The model under review builds one solid part; all positions refer to its coordinate system, in mm. A direction names the side the tool comes from. Round coordinates to 2 decimals unless told otherwise and drop trailing zeros. Write each loop counter-clockwise with the first axis right and the second up, starting at its lowest first coordinate (ties: lowest second). Pieces come first, ordered by that corner, then holes.
Item 1: Draft analysis for pull direction X (two halves, no side actions). For faces 3 (the face through (-2, 0, -32)), 4 (the face through (-21.623, -2.465, -175.575)), 5 (the face through (-4.51, -2.46, -138.88)), 6 (the face through (-126.15, -2.465, -55.314)), state which applies: +X half, -X half, draft (parallel to the pull), parting line (faces both ways), or undercut.
Item 2: Add section B-B (y = -3.9). State how many separate pieces and enclosed holes the cut face has, plus the area to 3 significant figures.
Item 3: To check wall thickness, follow L1, parallel to X at y = -1.05, z = -132.5; L2, parallel to X at y = -2.7, z = -132; L3, parallel to Z at x = 4.5, y = -4.1. State the ranges of each line that lie inside material, in increasing order.
Item 4: Machinability: for faces 1 (the face through (125.83, -2.46, -55.99)), 2 (the face through (20.94, -2.46, -175.7)), which of the approach directions +Z, -Z, +X, -X, +Y, -Y give a long, thin tool a straight path to every point of the face, cutting with its end or side? Answer none if there is none.
Item 5: Add section A-A (z = -162). Give the boundary of the cut face in (x, y), plus the area to 3 significant figures.
Item 6: Clearance check with flat-ended pins moving along their axes: pin 1 Ø2 at (x, y) = (55.5, -2.5) entering from +Z; pin 2 Ø1.5 at (y, z) = (-3, -121.5) entering from -X; pin 3 Ø2.5 at (y, z) = (-3.5, 6) entering from -X. State where each tip first meets the part, or that it passes through.
```python
from build123d import *

# Parameters (mm, degrees)
F0_R     = 1.6
F0_R_2   = 1.5
F1_DEPTH = 5


with BuildPart() as f1:
    # F0 (on Front) → F1 (new body)
    with BuildSketch(Plane.XZ):
        with BuildLine():
            Line((0, -105.5724638663), (0, -98.9320270717))
            Line((0, -98.9320270717), (0, -87.6365141757))
            Line((0, -87.6365141757), (-49.5, -87.6365141757))
            Line((-49.5, -87.6365141757), (-49.5, -59.3522429283))
            Line((-49.5, -59.3522429283), (0, -59.3522429283))
            Line((0, -59.3522429283), (0, 98.9320270717))
            add(Edge.make_bspline(
                [(-146.2381845713, 48.9320270717), (-143.2091262015, 68.9096288331), (-135.5852518703, 119.1915008468), (-50.9865840375, 106.55056484), (0, 98.9320270717)],
                knots=[0, 0, 0, 0, 0.3973122114, 1, 1, 1, 1], degree=3))
            Line((-146.2381845713, 48.9320270717), (-125, 48.9320270717))
            Line((-125, 48.9320270717), (-76.2381845713, 48.9320270717))
            Line((-76.2381845713, 48.9320270717), (-76.2381845713, -34.5724638663))
            Line((-76.2381845713, -34.5724638663), (-141.8916900928, -34.5724638663))
            ThreePointArc((-141.8916900928, -34.5724638663), (-125.9898971587, -55.6502114599), (-119.7161859861, -81.2974142364))
            Line((-119.7161859861, -81.2974142364), (-125, -98.9320270717))
            Line((-125, -98.9320270717), (-125, -142.2410042337))
            ThreePointArc((-125, -142.2410042337), (-123.6989053151, -148.3516501216), (-120.0213342443, -153.4022254914))
            Line((-120.0213342443, -153.4022254914), (-103.4289673704, -168.3000265931))
            ThreePointArc((-103.4289673704, -168.3000265931), (-65.4068612322, -117.6788317827), (-43.2242829938, -176.9757047349))
            ThreePointArc((-43.2242829938, -176.9757047349), (-44.2540337338, -178.1193368484), (-45.3315999714, -179.2180324392))
            ThreePointArc((-45.3315999714, -179.2180324392), (-21.2811980726, -175.6350274134), (0, -187.3981207609))
            Line((0, -187.3981207609), (0, -179.2180324392))
            Line((0, -179.2180324392), (0, -145.0724638663))
            ThreePointArc((0, -145.0724638663), (-1.0813916472, -144.6119791886), (-1.4988309156, -143.51325334))
            ThreePointArc((-1.4988309156, -143.51325334), (-16.4544826719, -134.0724638663), (-17.1526203097, -116.4000947784))
            ThreePointArc((-17.1526203097, -116.4000947784), (-17.7535207776, -114.3224638663), (-15.6537893941, -113.8040434806))
            ThreePointArc((-15.6537893941, -113.8040434806), (-8.843076746, -107.755805647), (0, -105.5724638663))
        make_face()
        with Locations((-59.6421356237, -73.494378552)):
            Circle(F0_R, mode=Mode.SUBTRACT)
        with BuildLine():
            ThreePointArc((-70.2381845713, -6.0724638663), (-71.298844743, -3.5118036945), (-68.7381845713, -4.5724638663))
            ThreePointArc((-68.7381845713, -4.5724638663), (-69.1775243995, -5.6331240381), (-70.2381845713, -6.0724638663))
        make_face(mode=Mode.SUBTRACT)
        with Locations((-64.1868777356, -4.5724638663)):
            Circle(F0_R_2, mode=Mode.SUBTRACT)
        with Locations((-58.2381845713, -4.5724638663)):
            Circle(F0_R_2, mode=Mode.SUBTRACT)
        with Locations((-70.2381845713, 24.4275361337)):
            Circle(F0_R_2, mode=Mode.SUBTRACT)
        with Locations((-64.2381845713, 24.4275361337)):
            Circle(F0_R_2, mode=Mode.SUBTRACT)
        with Locations((-58.2381845713, 24.4275361337)):
            Circle(F0_R_2, mode=Mode.SUBTRACT)
        with BuildLine():
            Line((0, -87.6365141757), (0, -98.9320270717))
            Line((0, -98.9320270717), (0, -105.5724638663))
            ThreePointArc((0, -105.5724638663), (8.843076746, -107.755805647), (15.6537893941, -113.8040434806))
            ThreePointArc((15.6537893941, -113.8040434806), (17.178692615, -113.7588733828), (17.9544826719, -115.0724638663))
            ThreePointArc((17.9544826719, -115.0724638663), (17.738462122, -115.8479616237), (17.1526203097, -116.4000947784))
            ThreePointArc((17.1526203097, -116.4000947784), (18.5324011651, -120.3831790756), (19, -124.5724638663))
            ThreePointArc((19, -124.5724638663), (13.9548878067, -137.4666915013), (1.4988309156, -143.51325334))
            ThreePointArc((1.4988309156, -143.51325334), (1.4997077004, -143.542852833), (1.5, -143.5724638663))
            ThreePointArc((1.5, -143.5724638663), (1.0606601718, -144.6331240381), (0, -145.0724638663))
            Line((0, -145.0724638663), (0, -179.2180324392))
            Line((0, -179.2180324392), (0, -187.3981207609))
            ThreePointArc((0, -187.3981207609), (21.2811980726, -175.6350274134), (45.3315999714, -179.2180324392))
            ThreePointArc((45.3315999714, -179.2180324392), (44.2540337338, -178.1193368484), (43.2242829938, -176.9757047349))
            ThreePointArc((43.2242829938, -176.9757047349), (65.4068612322, -117.6788317827), (103.4289673704, -168.3000265931))
            Line((103.4289673704, -168.3000265931), (120.0213342443, -153.4022254914))
            ThreePointArc((120.0213342443, -153.4022254914), (123.6989053151, -148.3516501216), (125, -142.2410042337))
            Line((125, -142.2410042337), (125, -98.9320270717))
            Line((125, -98.9320270717), (119.7161859861, -81.2974142364))
            ThreePointArc((119.7161859861, -81.2974142364), (125.9898971587, -55.6502114599), (141.8916900928, -34.5724638663))
            Line((141.8916900928, -34.5724638663), (76.2381845713, -34.5724638663))
            Line((76.2381845713, -34.5724638663), (76.2381845713, 48.9320270717))
            Line((76.2381845713, 48.9320270717), (125, 48.9320270717))
            Line((125, 48.9320270717), (146.2381845713, 48.9320270717))
            add(Edge.make_bspline(
                [(146.2381845713, 48.9320270717), (143.2091262015, 68.9096288331), (135.5852518703, 119.1915008468), (50.9865840375, 106.55056484), (0, 98.9320270717)],
                knots=[0, 0, 0, 0, 0.3973122114, 1, 1, 1, 1], degree=3))
            Line((0, 98.9320270717), (0, -59.3522429283))
            Line((0, -59.3522429283), (49.5, -59.3522429283))
            Line((49.5, -59.3522429283), (49.5, -87.6365141757))
            Line((49.5, -87.6365141757), (0, -87.6365141757))
        make_face()
        with Locations((59.6421356237, -73.494378552)):
            Circle(F0_R, mode=Mode.SUBTRACT)
        with Locations((58.2381845713, -4.5724638663)):
            Circle(F0_R_2, mode=Mode.SUBTRACT)
        with Locations((64.1868777356, -4.5724638663)):
            Circle(F0_R_2, mode=Mode.SUBTRACT)
        with Locations((70.2381845713, -4.5724638663)):
            Circle(F0_R_2, mode=Mode.SUBTRACT)
        with Locations((58.2381845713, 24.4275361337)):
            Circle(F0_R_2, mode=Mode.SUBTRACT)
        with Locations((64.2381845713, 24.4275361337)):
            Circle(F0_R_2, mode=Mode.SUBTRACT)
        with Locations((70.2381845713, 24.4275361337)):
            Circle(F0_R_2, mode=Mode.SUBTRACT)
        with BuildLine():
            ThreePointArc((15.6537893941, -113.8040434806), (8.843076746, -107.755805647), (0, -105.5724638663))
            Line((0, -105.5724638663), (0, -109.5724638663))
            ThreePointArc((0, -109.5724638663), (10.6066017178, -113.9658621485), (15, -124.5724638663))
            ThreePointArc((15, -124.5724638663), (10.6066017178, -135.1790655841), (0, -139.5724638663))
            Line((0, -139.5724638663), (0, -142.0724638663))
            ThreePointArc((0, -142.0724638663), (1.0395153223, -142.4910722191), (1.4988309156, -143.51325334))
            ThreePointArc((1.4988309156, -143.51325334), (13.9548878067, -137.4666915013), (19, -124.5724638663))
            ThreePointArc((19, -124.5724638663), (18.5324011651, -120.3831790756), (17.1526203097, -116.4000947784))
            ThreePointArc((17.1526203097, -116.4000947784), (15.1554445662, -115.8224638663), (15.6537893941, -113.8040434806))
        make_face()
        with BuildLine():
            Line((0, -109.5724638663), (0, -105.5724638663))
            ThreePointArc((0, -105.5724638663), (-8.843076746, -107.755805647), (-15.6537893941, -113.8040434806))
            ThreePointArc((-15.6537893941, -113.8040434806), (-15.1408921884, -114.3482539232), (-14.9544826719, -115.0724638663))
            ThreePointArc((-14.9544826719, -115.0724638663), (-15.6789849146, -116.3564433165), (-17.1526203097, -116.4000947784))
            ThreePointArc((-17.1526203097, -116.4000947784), (-16.4544826719, -134.0724638663), (-1.4988309156, -143.51325334))
            ThreePointArc((-1.4988309156, -143.51325334), (-1.0395153223, -142.4910722191), (0, -142.0724638663))
            Line((0, -142.0724638663), (0, -139.5724638663))
            ThreePointArc((0, -139.5724638663), (-15, -124.5724638663), (0, -109.5724638663))
        make_face()
    extrude(amount=F1_DEPTH)


solid = f1.part
```
Numbers:
1. face 3: draft
1. face 4: undercut
1. face 5: undercut
1. face 6: -X half
2. separate pieces: 1
2. enclosed holes: 19
2. area: 52,200 mm2
3. L1: x = -125 to -99.98, -41.13 to -12.73, 12.73 to 41.13, 99.98 to 125
3. L2: x = -125 to -99.62, -41.49 to -13.03, 13.03 to 41.49, 99.62 to 125
3. L3: z = -183.2 to -138.88, -110.26 to -87.64, -59.35 to 99.6
4. face 1: +X, +Y, -Y
4. face 2: -Z, +Y, -Y
5. outline: (-110.45, -5) - (-105.61, -5) - (-105.61, 0) - (-110.45, 0) - close; (-35.5, -5) - (35.5, -5) - (35.5, 0) - (-35.5, 0) - close; (105.61, -5) - (110.45, -5) - (110.45, 0) - (105.61, 0) - close
5. area: 403 mm2
6. pin 1: stops at z = 106.35
6. pin 2: stops at x = -125
6. pin 3: stops at x = -76.24
